For this review, take the finished solid that the model builds, in its own axes (mm). Coordinates: 2 decimals unless noted, no trailing zeros. Loops run counter-clockwise (first coordinate to the right, second up) from the corner with the lowest first, then second, coordinate; pieces in that order, holes last. Notation, with made-up numbers: (-7, 24) - (-3, 24) arc R20 ccw to (-3, 58) - close; hole circle Ø10 at (3, 21). An arc over 180 degrees is marked (long way). One line per item, written item: value. Start each with the question number.
1. Insertion check: pin 1 (1 mm diameter, centred on x = -22.5, y = -11.5, fed in from +Z). The pin has a flat end and moves straight along its axis. Give the tip position at first contact, or say it passes through.
2. Take a section at B-B, the plane z = 19. State the section outline as (x, y) points.
3. Take a section at A-A, the plane x = -25.95. State the section outline as (y, z) points, and give its area (3 significant figures).
4. To check wall thickness, follow line 1 (Z direction, x = -25.55, y = -15.2); line 2 (Z direction, x = -25.1, y = -13.7); line 3 (Y direction, x = -24.15, z = 24.5). State the ranges of each line that lie inside material, in increasing order. Write a range as from..to.
5. Take a section at C-C, the plane x = -22.05. State the section outline as (y, z) points, and give its area (3 significant figures).
```python
from build123d import *

# Parameters (mm, degrees)
SKETCH1_R           = 2.5
BOSS_EXTRUDE1_DEPTH = 38.61
SKETCH2_R           = 1.55
BOSS_EXTRUDE2_DEPTH = 2
FILLET1_R           = 0.5
BOSS_EXTRUDE3_START = 2
SKETCH3_R           = 1.55
BOSS_EXTRUDE3_DEPTH = 2
FILLET2_R           = 0.5


with BuildPart() as part:
    # Sketch1 → Boss-Extrude1 (new body)
    with BuildSketch(Plane.XY):
        with Locations((-23.972717512, -13.578911998)):
            Circle(SKETCH1_R)
    extrude(amount=BOSS_EXTRUDE1_DEPTH)

    # Sketch2 → Boss-Extrude2 (add)
    with BuildSketch(Plane.XY.offset(38.61)):
        with Locations((-23.972717512, -13.578911998)):
            Circle(SKETCH2_R)
    extrude(amount=BOSS_EXTRUDE2_DEPTH)

    # Fillet1
    fillet1_edges = [part.edges().sort_by_distance(p)[0] for p in [
        (-25.522717512, -13.578911998, 40.61),
    ]]
    fillet(fillet1_edges, radius=FILLET1_R)

    # Sketch3 → Boss-Extrude3 (add)
    with BuildSketch(Plane(origin=(0, 0, 0), x_dir=(-1, 0, 0), z_dir=(0, 0, -1)).offset(BOSS_EXTRUDE3_START)):
        with Locations(Location((23.972717512, -13.578911998, 0), (0, 0, 180))):
            Circle(SKETCH3_R)
    extrude(amount=-BOSS_EXTRUDE3_DEPTH)

    # Fillet2
    fillet2_edges = [part.edges().sort_by_distance(p)[0] for p in [
        (-25.522717512, -13.578911998, -2),
    ]]
    fillet(fillet2_edges, radius=FILLET2_R)


solid = part.part
```
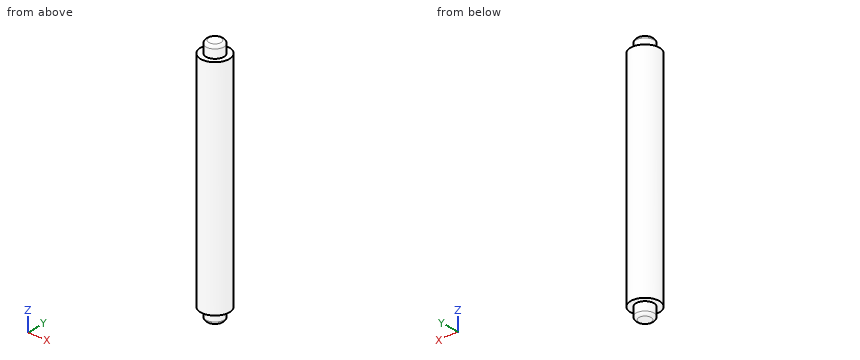
Solutions:
1. pin 1: z = 38.61
2. outline: circle Ø5 at (-23.97, -13.58)
3. outline: (-15.11, 0) - (-12.05, 0) - (-12.05, 38.61) - (-15.11, 38.61) - close
3. area: 118 mm2
4. line 1: 0..38.61
4. line 2: -1.99..40.6
4. line 3: -16.07..-11.09
5. outline: (-15.18, 0) - (-11.98, 0) - (-11.98, 38.61) - (-15.18, 38.61) - close
5. area: 123 mm2
